The model under review builds one solid part; all positions refer to its coordinate system, in mm. A direction names the side the tool comes from. Give positions to 0.01 mm unless a question says otherwise; leave off trailing zeros. Order: outer loops, then holes, each group sorted by start corner. A loop starts at its lowest first (then second) coordinate and runs counter-clockwise, first axis right, second up. Notation, with made-up numbers: (62.25, 14) - (90.25, 14) arc R22 cw to (90.25, 50) - close; hole circle Ø10 at (-24, -32). An arc over 180 degrees is marked (long way). Write item = value, one per line. Start each with the question number.
1. We need section D-D, the plane z = 3.5. Give the boundary of the cut face in (x, y) (3 decimals).
2. Mouldability with a two-part tool opening along Z and no side actions: class faces 6 (the flat face through (6.35, 1, 10)), 7 (the flat face through (-6.35, 1, 10)), 8 (the flat face through (0, 0, 0)), 9 (the cylindrical face through (-10.593, 11.455, 2.504)) as pulls with the +Z half, pulls with the -Z half, needs draft (parallel to the pull), parting line crosses it, or undercut.
3. We need section A-A, the plane z = 15.24. Give the boundary of the cut face in (x, y) (3 decimals), and give its area (3 significant figures).
4. For P1, Ø2.5, axis at y = -1, z = 10.5, coming from the +X side (3 decimals); P2, Ø5.5, axis at y = 1, z = 9, coming from the -X side (3 decimals); P3, Ø8, axis at y = 10, z = 7.5, coming from the +X side (3 decimals); P4, Ø2.5, axis at x = -0.5, z = 9, coming from the -Y side, all flat-tipped, find the tip position at first contact; note any pin that passes through.
5. Machinability: for faces 1 (the flat face through (-9.525, 3, 11)), 2 (the flat face through (3.175, -2, 15)), 3 (the cylindrical face through (14.79, 14.73, 2.5)), 4 (the flat face through (0, 1, 7.62)), 5 (the flat face through (9.525, 3, 11)), which of the approach directions +Z, -Z, +X, -X, +Y, -Y give a long, thin tool a straight path to every point of the face, cutting with its end or side? Answer none if there is none.
6. We need section B-B, the plane y = -2. Give the boundary of the cut face in (x, z) (3 decimals).
7. We need section C-C, the plane x = -2. Give the boundary of the cut face in (y, z) (3 decimals), and give its area (3 significant figures).
8. Wall thickness on probe 1 along X at (y, z) = (-1.5, 9.75) (3 decimals); probe 2 along Y at (x, z) = (4.5, 9.75) (3 decimals); probe 3 along Y at (x, z) = (9, 7.25) (3 decimals): over which ranges is each line inside the solid? List them lowest first.
from build123d import *

# Parameters (mm, degrees)
F0_R     = 1.593679
F1_DEPTH = 5.08
F2_W     = 19.05
F2_H     = 12.7
F3_DEPTH = 12.7
F4_W     = 6.35
F4_H     = 5.08
F5_DEPTH = 3.175
F6_W     = 12.7
F6_H     = 5.08
F7_DEPTH = 5.08
F8_R     = 1.27
F9_DEPTH = 12.7


with BuildPart() as f1:
    # F0 (on Top) → F1 (new body)
    with BuildSketch(Plane.XY):
        with BuildLine():
            ThreePointArc((15.875, 12.065), (14.759077, 14.759077), (12.065, 15.875))
            Line((12.065, 15.875), (-12.065, 15.875))
            ThreePointArc((-12.065, 15.875), (-14.759077, 14.759077), (-15.875, 12.065))
            Line((-15.875, 12.065), (-15.875, -12.065))
            ThreePointArc((-15.875, -12.065), (-14.759077, -14.759077), (-12.065, -15.875))
            Line((-12.065, -15.875), (12.065, -15.875))
            ThreePointArc((12.065, -15.875), (14.759077, -14.759077), (15.875, -12.065))
            Line((15.875, -12.065), (15.875, 12.065))
        make_face()
        with Locations((-12.065, -12.065)):
            Circle(F0_R, mode=Mode.SUBTRACT)
        with Locations((12.065, -12.065)):
            Circle(F0_R, mode=Mode.SUBTRACT)
        with Locations((-12.065, 12.065)):
            Circle(F0_R, mode=Mode.SUBTRACT)
        with Locations((12.065, 12.065)):
            Circle(F0_R, mode=Mode.SUBTRACT)
    extrude(amount=F1_DEPTH)

    # F2 (on face) → F3 (join)
    with BuildSketch(Plane.XY.offset(5.08)):
        with Locations((0, 3.175)):
            Rectangle(F2_W, F2_H)
    extrude(amount=F3_DEPTH)

    # F4 (on face) → F5 (cut)
    with BuildSketch(Plane.XZ.offset(3.175)):
        with Locations((0, 15.24)):
            Rectangle(F4_W, F4_H)
        Polygon((3.175, 12.7), (-3.175, 12.7), (-6.35, 12.7), (-6.35, 7.62), (6.35, 7.62), (6.35, 12.7), align=None)
    extrude(amount=-F5_DEPTH, mode=Mode.SUBTRACT)

    # F6 (on face) → F7 (cut)
    with BuildSketch(Plane.XZ):
        with Locations((0, 10.16)):
            Rectangle(F6_W, F6_H)
    extrude(amount=-F7_DEPTH, mode=Mode.SUBTRACT)

    # F8 (on face) → F9 (cut)
    with BuildSketch(Plane.XZ.offset(3.175)):
        with Locations((-6.35, 15.24)):
            Circle(F8_R)
        with Locations((6.35, 15.24)):
            Circle(F8_R)
    extrude(amount=-F9_DEPTH, mode=Mode.SUBTRACT)


solid = f1.part
Model answer:
q1.outline = (-15.875, -12.065) arc R3.81 ccw to (-12.065, -15.875) - (12.065, -15.875) arc R3.81 ccw to (15.875, -12.065) - (15.875, 12.065) arc R3.81 ccw to (12.065, 15.875) - (-12.065, 15.875) arc R3.81 ccw to (-15.875, 12.065) - close; hole circle Ø3.187 at (-12.065, -12.065); hole circle Ø3.187 at (-12.065, 12.065); hole circle Ø3.187 at (12.065, -12.065); hole circle Ø3.187 at (12.065, 12.065)
q2.face_6 = undercut
q2.face_7 = undercut
q2.face_8 = pulls with the -Z half
q2.face_9 = needs draft
q3.outline = (-9.525, -3.175) - (-7.62, -3.175) - (-7.62, 9.525) - (-9.525, 9.525) - close; (-5.08, -3.175) - (-3.175, -3.175) - (-3.175, 0) - (3.175, 0) - (3.175, -3.175) - (5.08, -3.175) - (5.08, 9.525) - (-5.08, 9.525) - close; (7.62, -3.175) - (9.525, -3.175) - (9.525, 9.525) - (7.62, 9.525) - close
q3.area = 157 mm2
q4.P1 = 9.525
q4.P2 = -9.525
q4.P3 = 15.875
q4.P4 = 5.08
q5.face_1 = +Z, -X, +Y, -Y
q5.face_2 = +Z, -Y
q5.face_3 = +Z, -Z, +X, +Y
q5.face_4 = -Y
q5.face_5 = +Z, +X, +Y, -Y
q6.outline = (-15.875, 0) - (15.875, 0) - (15.875, 5.08) - (9.525, 5.08) - (9.525, 17.78) - (3.175, 17.78) - (3.175, 12.7) - (6.35, 12.7) - (6.35, 7.62) - (-6.35, 7.62) - (-6.35, 12.7) - (-3.175, 12.7) - (-3.175, 17.78) - (-9.525, 17.78) - (-9.525, 5.08) - (-15.875, 5.08) - close; hole circle Ø2.54 at (-6.35, 15.24); hole circle Ø2.54 at (6.35, 15.24)
q7.outline = (-15.875, 0) - (15.875, 0) - (15.875, 5.08) - (9.525, 5.08) - (9.525, 17.78) - (0, 17.78) - (0, 12.7) - (5.08, 12.7) - (5.08, 7.62) - (-3.175, 7.62) - (-3.175, 5.08) - (-15.875, 5.08) - close
q7.area = 265 mm2
q8.probe_1 = -9.525 to -6.35, 6.35 to 9.525
q8.probe_2 = 5.08 to 9.525
q8.probe_3 = -3.175 to 9.525
